Could you check a few things on this model? Use its own coordinates, in mm. A direction names the side the tool comes from. Give positions to 0.01 mm unless a question says otherwise; leave off trailing zeros. Loops run counter-clockwise (first coordinate to the right, second up) from the corner with the lowest first, then second, coordinate; pieces in that order, holes last. Notation, with made-up numbers: M -32,84.5 L 5,84.5 A4 cw 5,91.5 Z; hole C 12.5,-10 d2. An arc over 180 degrees is marked long. Use a Markdown table: item, result. Add a question column.
1) If I drill on line 1 along Y through (x, z) = (0.5, 1.25); line 2 along X through (y, z) = (-14, 0.2); line 3 along Y through (x, z) = (-43.5, 2.2), over which ranges is the centre line in solid material (lowest first)? Write a range as [from, to].
2) Which directions (+Z, -Z, +X, -X, +Y, -Y) give clear straight access to the entire face, cutting with the end or side of a thin tool? Please do faces 1 (the flat face through (-27.126, -10.126, 2.535)), 2 (the flat face through (3, -82.887, 2)), 3 (the flat face through (-90, -93, 3)).
3) Will these pins go through, and if not, where does the flat tip stop? pin 1 Ø2.5 at (y, z) = (-7.5, 3.5) entering from +X; pin 2 Ø2.5 at (x, z) = (1.5, 2) entering from -Y; pin 3 Ø1.5 at (y, z) = (-8, 1.5) entering from -X.
4) We'd pull the mould along X, two halves only. Please class faces 4 (the flat face through (5, -33, 2)), 5 (the flat face through (-18, -7, 3)), 6 (the flat face through (-54, -104, 3)), 7 (the flat face through (-27.13, -105.02, 1.23)): +X half, -X half, draft (parallel to the pull), parting line (faces both ways), or undercut.
5) Suppose I cut it at B-B on y = -53. List the corners of the cut face in (x, z) for me.
6) Suppose I cut it at A-A on x = -25. List the corners of the cut face in (y, z) for me, and give its area (3 significant figures).
7) Suppose I cut it at C-C on x = -77. List the corners of the cut face in (y, z) for me, and give its area (3 significant figures).
```python
from build123d import *

# Parameters (mm, degrees)
ESQUISSE1_W                    = 90
ESQUISSE1_H                    = 100
BOSS_EXTRU_3_DEPTH             = 5
ENL_V_MAT_EXTRU_3_DEPTH        = 135.629120178
BOSS_EXTRU_4_DEPTH             = 90
ESQUISSE7_W                    = 18
ESQUISSE7_H                    = 5.773502692
ENL_V_MAT_EXTRU_4_DEPTH        = 137.787000854
ESQUISSE8_W                    = 18
ESQUISSE8_H                    = 5
ENL_V_MAT_EXTRU_5_DEPTH        = 133.498992691
ESQUISSE9_W                    = 18
ESQUISSE9_H                    = 5
ENL_V_MAT_EXTRU_6_DEPTH        = 133.498992691
BOSS_EXTRU_5_REACH             = 118.304
BOSS_EXTRU_5_DIRECTION_2_REACH = 118.304
ESQUISSE11_W                   = 18
ESQUISSE11_H                   = 13
BOSS_EXTRU_6_DEPTH             = 5
ENL_V_MAT_EXTRU_7_DEPTH        = 135.082064423
ESQUISSE13_W                   = 5
ESQUISSE13_H                   = 20
BOSS_EXTRU_7_DEPTH             = 5


with BuildPart() as part:
    # Esquisse1 → Boss.-Extru.3 (new body)
    with BuildSketch(Plane.XY):
        with Locations((-45, -50)):
            Rectangle(ESQUISSE1_W, ESQUISSE1_H)
    extrude(amount=BOSS_EXTRU_3_DEPTH)

    # Esquisse5 → Enlèv. mat.-Extru.3 (cut, through all)
    with BuildSketch(Plane(origin=(0, 0, 0), x_dir=(0, 0, -1), z_dir=(1, 0, 0))):
        Polygon((0, 0), (-5, 0), (-5, -5.773502692), (0, -2.886751346), align=None)
    extrude(amount=-ENL_V_MAT_EXTRU_3_DEPTH, mode=Mode.SUBTRACT)

    # Esquisse6 → Boss.-Extru.4 (add, through all)
    with BuildSketch(Plane(origin=(0, 0, 0), x_dir=(0, 0, -1), z_dir=(1, 0, 0))):
        Polygon((0, -100), (-5, -100), (0, -102.886751346), align=None)
    extrude(amount=-BOSS_EXTRU_4_DEPTH)

    # Esquisse7 → Enlèv. mat.-Extru.4 (cut, through all)
    with BuildSketch(Plane.XY.offset(5)):
        with Locations((-63, -8.660254038)):
            Rectangle(ESQUISSE7_W, ESQUISSE7_H)
        with Locations((-27, -8.660254038)):
            Rectangle(ESQUISSE7_W, ESQUISSE7_H)
    extrude(amount=-ENL_V_MAT_EXTRU_4_DEPTH, mode=Mode.SUBTRACT)

    # Esquisse8 → Enlèv. mat.-Extru.5 (cut, through all)
    with BuildSketch(Plane.XZ.offset(5.773502692)):
        with Locations((-63, 2.5)):
            Rectangle(ESQUISSE8_W, ESQUISSE8_H)
    extrude(amount=-ENL_V_MAT_EXTRU_5_DEPTH, mode=Mode.SUBTRACT)

    # Esquisse9 → Enlèv. mat.-Extru.6 (cut, through all)
    with BuildSketch(Plane.XZ.offset(5.773502692)):
        with Locations((-27, 2.5)):
            Rectangle(ESQUISSE9_W, ESQUISSE9_H)
    extrude(amount=-ENL_V_MAT_EXTRU_6_DEPTH, mode=Mode.SUBTRACT)

    # Esquisse10 → Boss.-Extru.5 (add, up to next)
    with BuildSketch(Plane(origin=(-36, 0, 0), x_dir=(0, 0, -1), z_dir=(1, 0, 0)), mode=Mode.PRIVATE) as boss_extru_5_sk1:
        Polygon((0, -11.547005384), (-5, -11.547005384), (0, -8.66380151), align=None)
    boss_extru_5_tool1 = extrude(boss_extru_5_sk1.sketch, amount=-BOSS_EXTRU_5_REACH, mode=Mode.PRIVATE) - part.part
    add(boss_extru_5_tool1.solids().sort_by_distance((-36, -10.585937, 1.666667))[0])

    # Esquisse10 → Boss.-Extru.5 direction 2 (add, up to next)
    with BuildSketch(Plane(origin=(-36, 0, 0), x_dir=(0, 0, -1), z_dir=(1, 0, 0)), mode=Mode.PRIVATE) as boss_extru_5_direction_2_sk1:
        Polygon((0, -11.547005384), (-5, -11.547005384), (0, -8.66380151), align=None)
    boss_extru_5_direction_2_tool1 = extrude(boss_extru_5_direction_2_sk1.sketch, amount=BOSS_EXTRU_5_DIRECTION_2_REACH, mode=Mode.PRIVATE) - part.part
    add(boss_extru_5_direction_2_tool1.solids().sort_by_distance((-36, -10.585937, 1.666667))[0])

    # Esquisse11 → Boss.-Extru.6 (add, through all)
    with BuildSketch(Plane.XY.offset(5)):
        with Locations((-63, -106.5)):
            Rectangle(ESQUISSE11_W, ESQUISSE11_H)
        with Locations((-27, -106.5)):
            Rectangle(ESQUISSE11_W, ESQUISSE11_H)
    extrude(amount=-BOSS_EXTRU_6_DEPTH)

    # Esquisse12 → Enlèv. mat.-Extru.7 (cut, through all)
    with BuildSketch(Plane.ZY.offset(72)):
        Polygon((0, -102.886751346), (2.5, -107.216878365), (5, -105.773502692), (5, -113), (0, -113), align=None)
    extrude(amount=-ENL_V_MAT_EXTRU_7_DEPTH, mode=Mode.SUBTRACT)

    # Esquisse13 → Boss.-Extru.7 (add, through all)
    with BuildSketch(Plane(origin=(0, 0, 0), x_dir=(-1, 0, 0), z_dir=(0, 0, -1))):
        with Locations((92.5, -32.886751346)):
            Rectangle(ESQUISSE13_W, ESQUISSE13_H)
        with Locations((92.5, -72.886751346)):
            Rectangle(ESQUISSE13_W, ESQUISSE13_H)
        with Locations((-2.5, -72.886751346)):
            Rectangle(ESQUISSE13_W, ESQUISSE13_H)
        with Locations((-2.5, -32.886751346)):
            Rectangle(ESQUISSE13_W, ESQUISSE13_H)
    extrude(amount=-BOSS_EXTRU_7_DEPTH)


solid = part.part
```
Answer block:
| question | item | result |
|---|---|---|
| 1 | line 1 | y = [-82.89, -62.89], [-42.89, -22.89] |
| 1 | line 2 | x = [-90, 0] |
| 1 | line 3 | y = [-101.62, -4.16] |
| 2 | face 1 | +Z, +Y |
| 2 | face 2 | +Z, -Z, +X, -Y |
| 2 | face 3 | +Z, -Z, -X, -Y |
| 3 | pin 1 | stops at x = 0 |
| 3 | pin 2 | stops at y = -82.89 |
| 3 | pin 3 | stops at x = -90 |
| 4 | face 4 | +X half |
| 4 | face 5 | undercut |
| 4 | face 6 | undercut |
| 4 | face 7 | draft |
| 5 | outline | M -90,0 L 0,0 L 0,5 L -90,5 Z |
| 6 | outline | M -107.22,2.5 L -102.89,0 L -8.66,0 L -11.55,5 L -105.77,5 Z |
| 6 | area | 478 mm^2 |
| 7 | outline | M -102.89,0 L -2.89,0 L -5.77,5 L -100,5 Z |
| 7 | area | 486 mm^2 |
